```python
from build123d import *

# Parameters (mm, degrees)
SKETCH1_R           = 16
SKETCH1_R_2         = 4
SKETCH1_R_3         = 6
BOSS_EXTRUDE1_DEPTH = 5
SKETCH7_R           = 2.6
CUT_EXTRUDE1_DEPTH  = 7
BOSS_EXTRUDE6_DEPTH = 8
SKETCH9_R           = 1.6
CUT_EXTRUDE2_DEPTH  = 6
SKETCH10_R          = 2.6
BOSS_EXTRUDE7_DEPTH = 5
CUT_EXTRUDE4_START  = -10
SKETCH12_R          = 2.6
CUT_EXTRUDE4_DEPTH  = 10
SKETCH11_R          = 1.1
CUT_EXTRUDE3_DEPTH  = 6


with BuildPart() as part:
    # Sketch1 → Boss-Extrude1 (new body)
    # profile 1 of 3: a face of its own
    with BuildSketch(Plane.XY):
        with BuildLine():
            ThreePointArc((-63.902777778, -26.586845234), (-84.375, 0), (-63.902777778, 26.586845234))
            Line((-63.902777778, 26.586845234), (-105.963888889, 15.468709954))
            ThreePointArc((-105.963888889, 15.468709954), (-92.113397217, 12.677188612), (-85.875, 0))
            ThreePointArc((-85.875, 0), (-92.113397217, -12.677188612), (-105.963888889, -15.468709954))
            Line((-105.963888889, -15.468709954), (-63.902777778, -26.586845234))
        make_face()
    # profile 2 of 3: a face of its own
    with BuildSketch(Plane.XY):
        with Locations((-101.875, 0)):
            Circle(SKETCH1_R)
        with Locations((-101.875, 0)):
            Circle(SKETCH1_R_2, mode=Mode.SUBTRACT)
    # profile 3 of 3: a face of its own
    with BuildSketch(Plane.XY):
        with BuildLine():
            Line((-58.265804598, 27.46480771), (50.206034483, 32.957769253))
            ThreePointArc((50.206034483, 32.957769253), (84.875, 0), (50.206034483, -32.957769253))
            Line((50.206034483, -32.957769253), (-58.265804598, -27.46480771))
            ThreePointArc((-58.265804598, -27.46480771), (-84.375, 0), (-58.265804598, 27.46480771))
        make_face()
        with Locations((51.875, 0)):
            Circle(SKETCH1_R_3, mode=Mode.SUBTRACT)
    extrude(amount=BOSS_EXTRUDE1_DEPTH)

    # Sketch7 → Cut-Extrude1 (cut)
    with BuildSketch(Plane.XY.offset(5)):
        with Locations((29.375, 0)):
            Circle(SKETCH7_R)
        with Locations((74.375, 0)):
            Circle(SKETCH7_R)
    extrude(amount=-CUT_EXTRUDE1_DEPTH, mode=Mode.SUBTRACT)

    # Sketch8 → Boss-Extrude6 (add)
    with BuildSketch(Plane.XY.offset(5)):
        Polygon((-26.375, 28.464101615), (-28.375, 25), (-26.375, 21.535898385), (-22.375, 21.535898385), (-20.375, 25), (-22.375, 28.464101615), align=None)
        Polygon((-25.991580754, 27.8), (-27.608161507, 25), (-25.991580754, 22.2), (-22.758419246, 22.2), (-21.141838493, 25), (-22.758419246, 27.8), align=None, mode=Mode.SUBTRACT)
    boss_extrude6 = extrude(amount=-BOSS_EXTRUDE6_DEPTH)

    # Sketch9 → Cut-Extrude2 (cut)
    with BuildSketch(Plane.XY.offset(5)):
        with Locations((-24.375, 25)):
            Circle(SKETCH9_R)
    cut_extrude2 = extrude(amount=-CUT_EXTRUDE2_DEPTH, mode=Mode.SUBTRACT)

    # Mirror1: Boss-Extrude6 across plane
    add(boss_extrude6.mirror(Plane.ZX))

    # Mirror2: Cut-Extrude2 across plane
    add(cut_extrude2.mirror(Plane.ZX), mode=Mode.SUBTRACT)

    # Sketch10 → Boss-Extrude7 (add)
    with BuildSketch(Plane.XY.offset(5)):
        with Locations((-36.06831441, 11.178241177)):
            Circle(SKETCH10_R)
        with Locations(Location((-64.742423683, 22.173717984, 0), (0, 0, 180))):
            Circle(SKETCH10_R)
        Polygon((-41.60537748, 11.695000918), (-60.279486753, 18.855841852), (-59.205360613, 21.656958243), (-40.53125134, 14.496117309), align=None)
    extrude(amount=BOSS_EXTRUDE7_DEPTH)

    # Sketch12 → Cut-Extrude4 (cut)
    with BuildSketch(Plane.XY.offset(10).offset(CUT_EXTRUDE4_START)):
        with Locations((-36.06831441, 11.178241177)):
            Circle(SKETCH12_R)
        with Locations((-64.742423683, 22.173717984)):
            Circle(SKETCH12_R)
        Polygon((-59.320493296, 21.915307745), (-40.272901838, 14.611249993), (-41.490244797, 11.436651416), (-60.537836255, 18.740709168), align=None)
    extrude(amount=CUT_EXTRUDE4_DEPTH, mode=Mode.SUBTRACT)

    # Sketch11 → Cut-Extrude3 (cut)
    with BuildSketch(Plane.XY.offset(5)):
        with Locations((-88.581577383, -3.513888889)):
            Circle(SKETCH11_R)
        with Locations((-115.168422617, 3.513888889)):
            Circle(SKETCH11_R)
    extrude(amount=-CUT_EXTRUDE3_DEPTH, mode=Mode.SUBTRACT)


solid = part.part
```
Could you check a few things on this model? Use its own coordinates, in mm. A direction names the side the tool comes from. Give positions to 0.01 mm unless a question says otherwise; leave off trailing zeros. Order: outer loops, then holes, each group sorted by start corner. A loop starts at its lowest first (then second) coordinate and runs counter-clockwise, first axis right, second up.
Q1. I'm going to push flat-ended pins straight in: P1, Ø2.5, axis at x = -88.58, y = -3.51, coming from the +Z side; P2, Ø6, axis at x = 74.375, y = 0, coming from the -Z side; P3, Ø1.5, axis at x = -23.5, z = -2, coming from the +Y side; P4, Ø2.5, axis at x = -24.5, z = -1.5, coming from the -Y side. Where does each tip first touch, or does it pass through?
Q2. Suppose I cut it at B-B, the plane x = 16. Write out the boundary of the cut face in (y, z).
Q3. We'd pull the mould along X, two halves only. Please class faces 1 (the cylindrical face through (26.778, 0.114, 2.535)), 2 (the flat face through (-22, 27, -3)), 3 (the cylindrical face through (-61.147, 27.166, 2.465)): +X half, -X half, draft (parallel to the pull), parting line (faces both ways), or undercut.
Q4. For faces 4 (the flat face through (-50.881, 15.038, 2.465)), 5 (the flat face through (-26, -24, 0)), 6 (the flat face through (-4.789, 30.173, 2.465)), which set-ups out of +Z, -Z, +X, -X, +Y, -Y let a thin tool reach every point of the face, with its end or its side?
Q5. Suppose I cut it at A-A, the plane y = 0. Write out the boundary of the cut face in (x, z) (3 decimals).
Q6. Suppose I cut it at C-C, the plane x = 38. Write out the boundary of the cut face in (y, z).
Q7. If I drill on line 1 along Z through (x, y) = (75, 13); line 2 along Y through (x, z) = (57, 4.5); line 3 along Y through (x, z) = (29, 1.25), over which ranges is the centre line in solid material (lowest first)?
Solution:
1. P1: stops at z = 5
1. P2: stops at z = 0
1. P3: stops at y = 28.46
1. P4: stops at y = -28.46
2. outline: (-31.23, 0) - (31.23, 0) - (31.23, 5) - (-31.23, 5) - close
3. face 1: undercut
3. face 2: draft
3. face 3: -X half
4. face 4: +Z, -Z
4. face 5: -Z
4. face 6: +Z, -Z, -X, +Y
5. outline: (-117.875, 0) - (-105.875, 0) - (-105.875, 5) - (-117.875, 5) - close; (-97.875, 0) - (26.775, 0) - (26.775, 5) - (-97.875, 5) - close; (31.975, 0) - (45.875, 0) - (45.875, 5) - (31.975, 5) - close; (57.875, 0) - (71.775, 0) - (71.775, 5) - (57.875, 5) - close; (76.975, 0) - (84.875, 0) - (84.875, 5) - (76.975, 5) - close
6. outline: (-32.34, 0) - (32.34, 0) - (32.34, 5) - (-32.34, 5) - close
7. line 1: z = 0 to 5
7. line 2: y = -32.6 to -3.12, 3.12 to 32.6
7. line 3: y = -31.88 to -2.57, 2.57 to 31.88
